Can you work these out from the drawing? Everything is in mm from the part's minimum corner. Coordinates: 2 decimals unless noted, no trailing zeros. Write each loop counter-clockwise with the first axis right and the second up, starting at its lowest first coordinate (ties: lowest second). Pieces come first, ordered by that corner, then holes. Notation, with made-up numbers: M 19.5,88.5 L 73.5,88.5 A13 ccw 73.5,110.5 Z; hole C -40,60.25 d5. An arc over 180 degrees is marked long. Use one line per item in the form item = value. Start each with the question number.
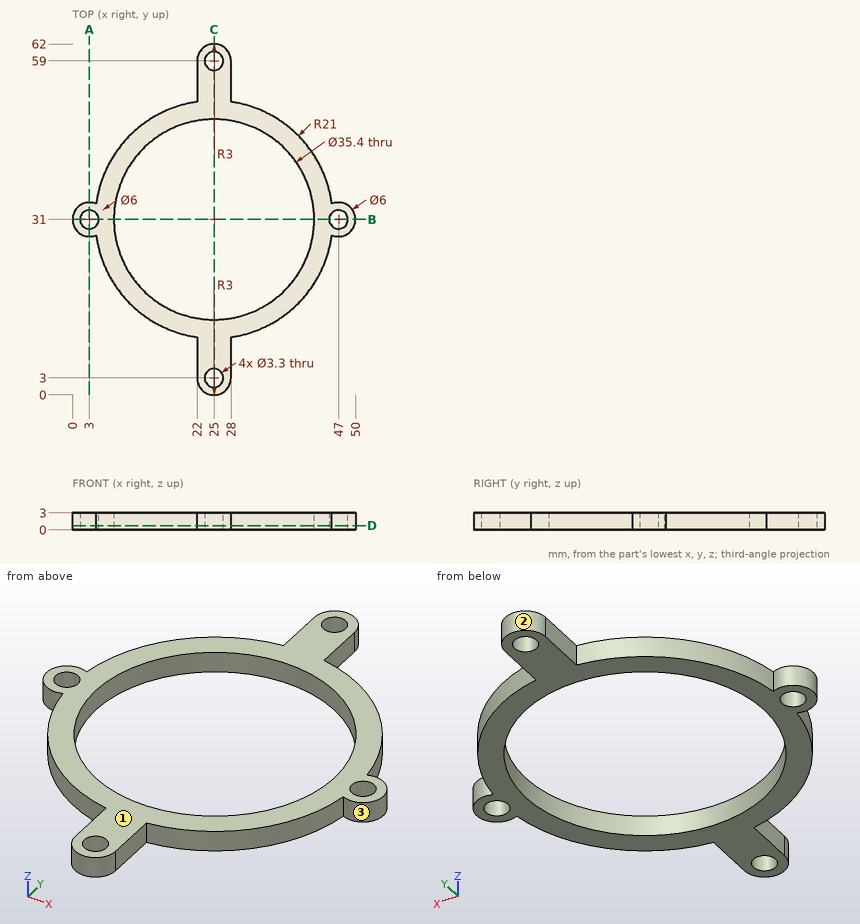
1) Suppose I cut it at B-B on y = 31. Please give me the cut outline in (x, z).
2) Suppose I cut it at A-A on x = 3. Please give me the cut outline in (y, z).
3) If we mould it in two halves opening along X, with no side actions, what happens to the marked faces 1, 2 and 3? For each: +X half, -X half, draft (parallel to the pull), parting line (faces both ways), or undercut.
4) Suppose I cut it at C-C on x = 25. Please give me the cut outline in (y, z).
5) Will these pins go through, and if not, where does the flat tip stop? pin 1 Ø1.5 at (y, z) = (55, 1) entering from -X; pin 2 Ø2 at (x, y) = (25, 59) entering from -Z; pin 3 Ø1.5 at (x, z) = (43.5, 1) entering from +Y.
6) Suppose I cut it at D-D on z = 0.75. Please give me the cut outline in (x, y), and give its area (3 significant figures).
7) Please list where these lines run through material, in increasing order: line 1 (Y direction, x = 25, z = 2.35); line 2 (Y direction, x = 47, z = 1.6); line 3 (X direction, y = 31.5, z = 2.3).
Computed values:
q1.outline = M 0,0 L 1.35,0 L 1.35,3 L 0,3 Z; M 4.65,0 L 7.3,0 L 7.3,3 L 4.65,3 Z; M 42.7,0 L 45.35,0 L 45.35,3 L 42.7,3 Z; M 48.65,0 L 50,0 L 50,3 L 48.65,3 Z
q2.outline = M 28,0 L 29.35,0 L 29.35,3 L 28,3 Z; M 32.65,0 L 34,0 L 34,3 L 32.65,3 Z
q3.face_1 = draft
q3.face_2 = parting line
q3.face_3 = undercut
q4.outline = M 0,0 L 1.35,0 L 1.35,3 L 0,3 Z; M 4.65,0 L 13.3,0 L 13.3,3 L 4.65,3 Z; M 48.7,0 L 57.35,0 L 57.35,3 L 48.7,3 Z; M 60.65,0 L 62,0 L 62,3 L 60.65,3 Z
q5.pin_1 = 22
q5.pin_2 = through
q5.pin_3 = 42.22
q6.outline = M 4.18,28.24 A21 ccw 22,10.22 L 22,3 A3 ccw 28,3 L 28,10.22 A21 ccw 45.82,28.24 A3 ccw long 45.82,33.76 A21 ccw 28,51.78 L 28,59 A3 ccw 22,59 L 22,51.78 A21 ccw 4.18,33.76 A3 ccw long Z; hole C 3,31 d3.3; hole C 25,31 d35.4; hole C 25,3 d3.3; hole C 25,59 d3.3; hole C 47,31 d3.3
q6.area = 521 mm²
q7.line_1 = 0 to 1.35, 4.65 to 13.3, 48.7 to 57.35, 60.65 to 62
q7.line_2 = 28 to 29.35, 32.65 to 34
q7.line_3 = 0.04 to 1.43, 4.57 to 7.31, 42.69 to 45.43, 48.57 to 49.96
